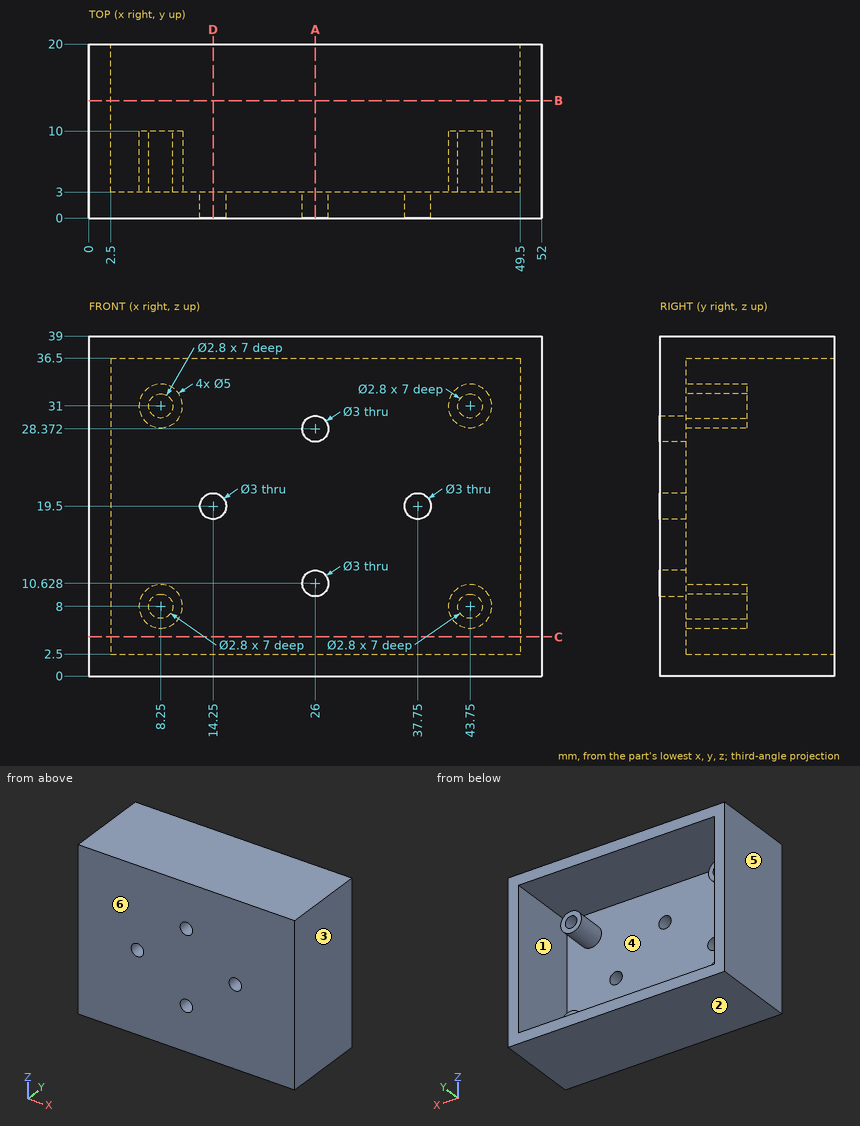
Part print with two shaded views. Sizes in mm from the minimum x, y, z corner. A direction names the side the tool comes from. Give positions to 0.01 mm unless a question says otherwise; leave off trailing zeros. Order: outer loops, then holes, each group sorted by start corner. A loop starts at its lowest first (then second) coordinate and runs counter-clockwise, first axis right, second up. Notation, with made-up numbers: M 62,12.5 L 116,12.5 A18 cw 116,32.5 Z; hole C -34.75,52.5 d8. An arc over 180 degrees is marked long. Use one line per item in the form item = value.
1) Drop flat-ended pins along their axis: pin 1 (4 mm diameter, centred on x = 37.75, z = 19.5, fed in from +Y); pin 2 (3.5 mm diameter, centred on x = 8.25, z = 31, fed in from +Y); pin 3 (2.5 mm diameter, centred on x = 26, z = 28.37, fed in from +Y). Give the stop position or say it passes through.
Calculated:
pin_1 = 3
pin_2 = 10
pin_3 = through
2) Saw through at B-B (y = 13.5). Give the cut face in (x, z), plus the area to 3 significant figures.
Calculated:
outline = M 0,0 L 52,0 L 52,39 L 0,39 Z; hole M 2.5,2.5 L 49.5,2.5 L 49.5,36.5 L 2.5,36.5 Z
area = 430 mm2
3) Saw through at C-C (z = 4.5). Give the cut face in (x, y), plus the area to 3 significant figures.
Calculated:
outline = M 0,0 L 52,0 L 52,20 L 49.5,20 L 49.5,3 L 2.5,3 L 2.5,20 L 0,20 Z
area = 241 mm2
4) Two-plate mould, pull along X, no slides. Class the marked faces 3, 4, 5 and 6: released by +X, released by -X, zero draft, split by the parting line, or undercut.
Calculated:
face_3 = released by +X
face_4 = undercut
face_5 = released by -X
face_6 = zero draft
5) Tool access for the marked faces 1 and 2: list every direction of +Z, -Z, +X, -X, +Y, -Y with a clear straight run to the whole face (end or side of a thin tool).
Calculated:
face_1 = +Y
face_2 = -Z, +X, -X, +Y, -Y
6) Saw through at A-A (x = 26). Give the cut face in (y, z), plus the area to 3 significant figures.
Calculated:
outline = M 0,0 L 20,0 L 20,2.5 L 3,2.5 L 3,9.13 L 0,9.13 Z; M 0,12.13 L 3,12.13 L 3,26.87 L 0,26.87 Z; M 0,29.87 L 3,29.87 L 3,36.5 L 20,36.5 L 20,39 L 0,39 Z
area = 184 mm2
7) Probe probe 1 along X at (y, z) = (4.75, 8); probe 2 along Z at (x, y) = (33, 5.75); probe 3 along Z at (x, y) = (14.25, 1.45). List the from-to ranges inside material, lowest first.
Calculated:
probe_1 = 0 to 2.5, 5.75 to 6.85, 9.65 to 10.75, 41.25 to 42.35, 45.15 to 46.25, 49.5 to 52
probe_2 = 0 to 2.5, 36.5 to 39
probe_3 = 0 to 18, 21 to 39
8) Saw through at D-D (x = 14.25). Give the cut face in (y, z), plus the area to 3 significant figures.
Calculated:
outline = M 0,0 L 20,0 L 20,2.5 L 3,2.5 L 3,18 L 0,18 Z; M 0,21 L 3,21 L 3,36.5 L 20,36.5 L 20,39 L 0,39 Z
area = 193 mm2
